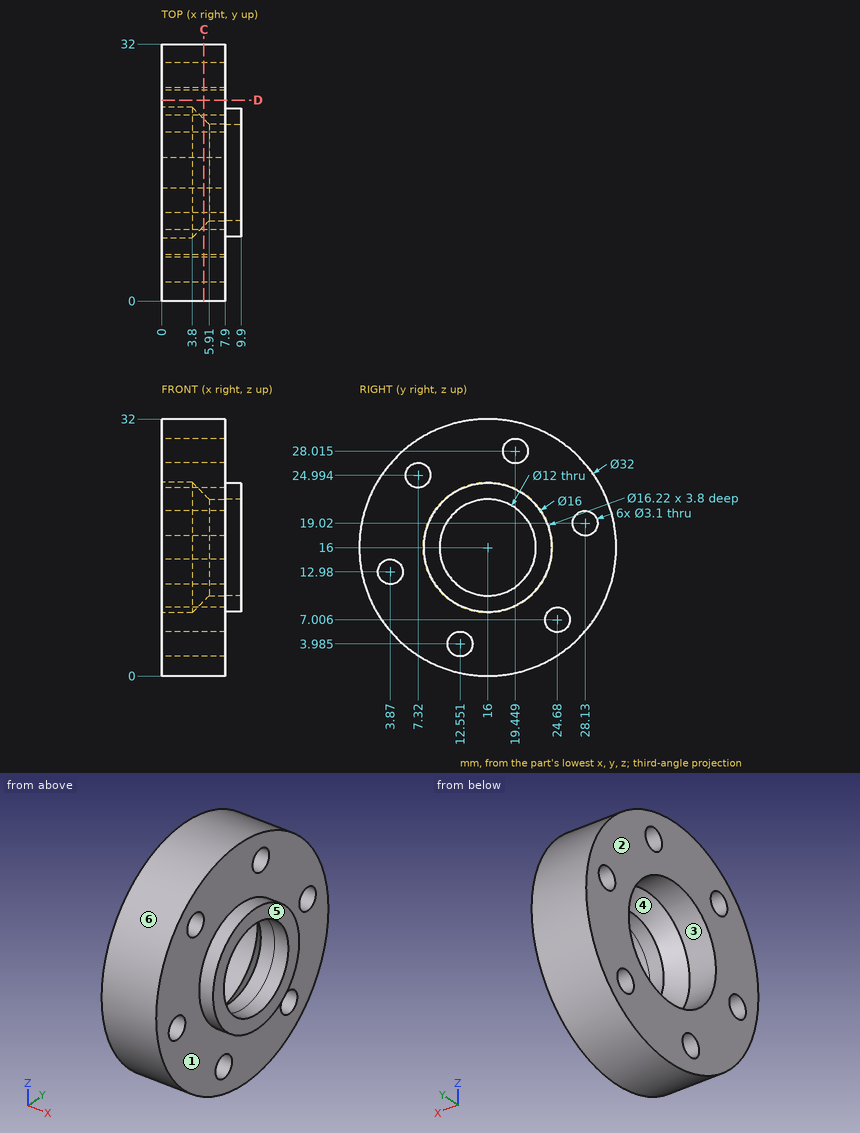
Part print with two shaded views. Sizes in mm from the minimum x, y, z corner. A direction names the side the tool comes from. Coordinates: 2 decimals unless noted, no trailing zeros. Order: outer loops, then holes, each group sorted by start corner. A loop starts at its lowest first (then second) coordinate and runs counter-clockwise, first axis right, second up. Notation, with made-up numbers: (16, 54.5) - (68, 54.5) arc R20 cw to (68, 68.5) - close; hole circle Ø10 at (57.5, -24.5). An arc over 180 degrees is marked (long way). Write item = value, one per line. Start each with the question number.
1) Saw through at C-C on x = 5.25. Count the separate pieces of the cut face and the enclosed holes in it.
2) Saw through at D-D on y = 25. Write the cut outline in (x, z).
3) Wall check: line 1 along Z through (x, y) = (1.4, 16); line 2 along Z through (x, y) = (4.5, 28) (1 decimal); line 3 along Y through (x, z) = (2.5, 19) (1 decimal). Give the ranges that are in metal, low to high. Write a range as from..to.
4) Two-plate mould, pull along Y, no slides. Class the marked faces 4, 5 and 6: pulls with the +Y half, pulls with the -Y half, needs draft (parallel to the pull), parting line crosses it, or undercut.
5) 3-axis set-ups, long thin cutter, end or side, ignore diameter. For the marked faces 1, 2 and 3: which of +Z, -Z, +X, -X, +Y, -Y reach the whole face in a straight line?
6) Flat gauge pins, fed straight in: pin 1 Ø1 at (y, z) = (23.5, 7) entering from +X; pin 2 Ø5 at (y, z) = (28.13, 19.02) entering from -X; pin 3 Ø4 at (x, y) = (6.5, 3.5) entering from +Z; pin 4 Ø3 at (x, y) = (1.5, 22) entering from +Z (1 decimal). Where does each tip first touch, or does it go through?
From the geometry:
q1.separate_pieces = 1
q1.enclosed_holes = 7
q2.outline = (0, 2.77) - (7.9, 2.77) - (7.9, 5.49) - (0, 5.49) - close; (0, 8.52) - (7.9, 8.52) - (7.9, 29.23) - (0, 29.23) - close
q3.line_1 = 0..7.89, 24.11..32
q3.line_2 = 5.4..17.5, 20.6..26.6
q3.line_3 = 0.3..8.5, 23.5..26.6, 29.7..31.7
q4.face_4 = undercut
q4.face_5 = needs draft
q4.face_6 = parting line crosses it
q5.face_1 = +X
q5.face_2 = +Z, -Z, -X, +Y, -Y
q5.face_3 = -X
q6.pin_1 = 7.9
q6.pin_2 = 0
q6.pin_3 = 28.07
q6.pin_4 = 31.4
